Here's how the part is built. I have some questions about the finished solid (model axes, mm). Coordinates: 2 decimals unless noted, no trailing zeros. Write each loop counter-clockwise with the first axis right and the second up, starting at its lowest first coordinate (ties: lowest second). Pieces come first, ordered by that corner, then holes. Notation, with made-up numbers: (-2, 35) -> (41, 35) arc R23 ccw to (41, 47) -> close; hole circle Ø3 at (20, 64). An arc over 180 degrees is marked (long way). Put each result on its own line as item: value. Start each with the question number.
Item 1: I want a section at B-B, the plane x = 150. List the corners of the cut face in (y, z) for me, then the cut area to 3 significant figures.
Item 2: I want a section at A-A, the plane y = 94.5. List the corners of the cut face in (x, z) for me, then the cut area to 3 significant figures.
Item 3: I need wall thicknesses on line 1 (X direction, y = 254.5, z = 1); line 2 (X direction, y = 205, z = 5.25); line 3 (Y direction, x = -48, z = 0.5). Which ranges of each line are inside material? Lowest first, please. Write a range as [from, to].
Item 4: I want a section at C-C, the plane z = 10. State how many separate pieces and enclosed holes the cut face has, then the cut area to 3 significant figures.
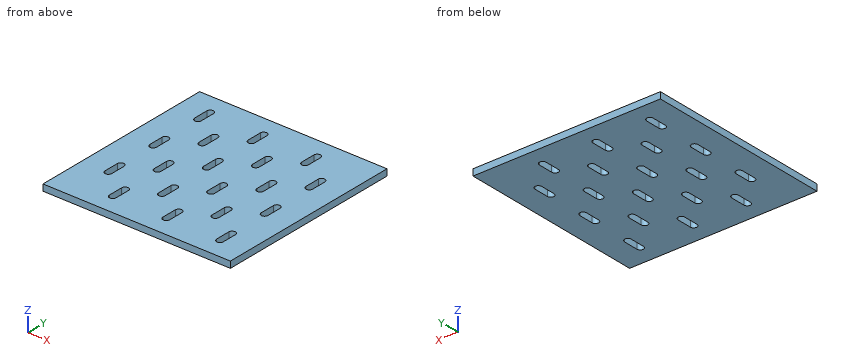
from build123d import *

# Parameters (mm, degrees)
SKETCH_1_W      = 350
SKETCH_1_H      = 350
EXTRUDE_1_DEPTH = 12


with BuildPart() as part:
    # Эскиз1 → Бобышка-Вытянуть1 (new body)
    with BuildSketch(Plane.XY):
        with Locations((75, 125)):
            Rectangle(SKETCH_1_W, SKETCH_1_H)
        with BuildLine():
            Line((6.25, 13.75), (6.25, -13.75))
            ThreePointArc((6.25, -13.75), (0, -20), (-6.25, -13.75))
            Line((-6.25, -13.75), (-6.25, 13.75))
            ThreePointArc((-6.25, 13.75), (0, 20), (6.25, 13.75))
        make_face(mode=Mode.SUBTRACT)
        with BuildLine():
            Line((-43.75, 63.75), (-43.75, 36.25))
            ThreePointArc((-43.75, 36.25), (-50, 30), (-56.25, 36.25))
            Line((-56.25, 36.25), (-56.25, 63.75))
            ThreePointArc((-56.25, 63.75), (-50, 70), (-43.75, 63.75))
        make_face(mode=Mode.SUBTRACT)
        with BuildLine():
            Line((106.25, 13.75), (106.25, -13.75))
            ThreePointArc((106.25, -13.75), (100, -20), (93.75, -13.75))
            Line((93.75, -13.75), (93.75, 13.75))
            ThreePointArc((93.75, 13.75), (100, 20), (106.25, 13.75))
        make_face(mode=Mode.SUBTRACT)
        with BuildLine():
            Line((56.25, 63.75), (56.25, 36.25))
            ThreePointArc((56.25, 36.25), (50, 30), (43.75, 36.25))
            Line((43.75, 36.25), (43.75, 63.75))
            ThreePointArc((43.75, 63.75), (50, 70), (56.25, 63.75))
        make_face(mode=Mode.SUBTRACT)
        with BuildLine():
            Line((206.25, 13.75), (206.25, -13.75))
            ThreePointArc((206.25, -13.75), (200, -20), (193.75, -13.75))
            Line((193.75, -13.75), (193.75, 13.75))
            ThreePointArc((193.75, 13.75), (200, 20), (206.25, 13.75))
        make_face(mode=Mode.SUBTRACT)
        with BuildLine():
            Line((156.25, 63.75), (156.25, 36.25))
            ThreePointArc((156.25, 36.25), (150, 30), (143.75, 36.25))
            Line((143.75, 36.25), (143.75, 63.75))
            ThreePointArc((143.75, 63.75), (150, 70), (156.25, 63.75))
        make_face(mode=Mode.SUBTRACT)
        with BuildLine():
            Line((106.25, 113.75), (106.25, 86.25))
            ThreePointArc((106.25, 86.25), (100, 80), (93.75, 86.25))
            Line((93.75, 86.25), (93.75, 113.75))
            ThreePointArc((93.75, 113.75), (100, 120), (106.25, 113.75))
        make_face(mode=Mode.SUBTRACT)
        with BuildLine():
            Line((56.25, 163.75), (56.25, 136.25))
            ThreePointArc((56.25, 136.25), (50, 130), (43.75, 136.25))
            Line((43.75, 136.25), (43.75, 163.75))
            ThreePointArc((43.75, 163.75), (50, 170), (56.25, 163.75))
        make_face(mode=Mode.SUBTRACT)
        with BuildLine():
            Line((206.25, 113.75), (206.25, 86.25))
            ThreePointArc((206.25, 86.25), (200, 80), (193.75, 86.25))
            Line((193.75, 86.25), (193.75, 113.75))
            ThreePointArc((193.75, 113.75), (200, 120), (206.25, 113.75))
        make_face(mode=Mode.SUBTRACT)
        with BuildLine():
            Line((156.25, 163.75), (156.25, 136.25))
            ThreePointArc((156.25, 136.25), (150, 130), (143.75, 136.25))
            Line((143.75, 136.25), (143.75, 163.75))
            ThreePointArc((143.75, 163.75), (150, 170), (156.25, 163.75))
        make_face(mode=Mode.SUBTRACT)
        with BuildLine():
            Line((106.25, 213.75), (106.25, 186.25))
            ThreePointArc((106.25, 186.25), (100, 180), (93.75, 186.25))
            Line((93.75, 186.25), (93.75, 213.75))
            ThreePointArc((93.75, 213.75), (100, 220), (106.25, 213.75))
        make_face(mode=Mode.SUBTRACT)
        with BuildLine():
            Line((56.25, 263.75), (56.25, 236.25))
            ThreePointArc((56.25, 236.25), (50, 230), (43.75, 236.25))
            Line((43.75, 236.25), (43.75, 263.75))
            ThreePointArc((43.75, 263.75), (50, 270), (56.25, 263.75))
        make_face(mode=Mode.SUBTRACT)
        with BuildLine():
            Line((206.25, 213.75), (206.25, 186.25))
            ThreePointArc((206.25, 186.25), (200, 180), (193.75, 186.25))
            Line((193.75, 186.25), (193.75, 213.75))
            ThreePointArc((193.75, 213.75), (200, 220), (206.25, 213.75))
        make_face(mode=Mode.SUBTRACT)
        with BuildLine():
            Line((156.25, 263.75), (156.25, 236.25))
            ThreePointArc((156.25, 236.25), (150, 230), (143.75, 236.25))
            Line((143.75, 236.25), (143.75, 263.75))
            ThreePointArc((143.75, 263.75), (150, 270), (156.25, 263.75))
        make_face(mode=Mode.SUBTRACT)
        with BuildLine():
            Line((6.25, 113.75), (6.25, 86.25))
            ThreePointArc((6.25, 86.25), (0, 80), (-6.25, 86.25))
            Line((-6.25, 86.25), (-6.25, 113.75))
            ThreePointArc((-6.25, 113.75), (0, 120), (6.25, 113.75))
        make_face(mode=Mode.SUBTRACT)
        with BuildLine():
            Line((-43.75, 163.75), (-43.75, 136.25))
            ThreePointArc((-43.75, 136.25), (-50, 130), (-56.25, 136.25))
            Line((-56.25, 136.25), (-56.25, 163.75))
            ThreePointArc((-56.25, 163.75), (-50, 170), (-43.75, 163.75))
        make_face(mode=Mode.SUBTRACT)
        with BuildLine():
            Line((6.25, 213.75), (6.25, 186.25))
            ThreePointArc((6.25, 186.25), (0, 180), (-6.25, 186.25))
            Line((-6.25, 186.25), (-6.25, 213.75))
            ThreePointArc((-6.25, 213.75), (0, 220), (6.25, 213.75))
        make_face(mode=Mode.SUBTRACT)
        with BuildLine():
            Line((-43.75, 263.75), (-43.75, 236.25))
            ThreePointArc((-43.75, 236.25), (-50, 230), (-56.25, 236.25))
            Line((-56.25, 236.25), (-56.25, 263.75))
            ThreePointArc((-56.25, 263.75), (-50, 270), (-43.75, 263.75))
        make_face(mode=Mode.SUBTRACT)
    extrude(amount=EXTRUDE_1_DEPTH)


solid = part.part
Calculated:
1. outline: (-50, 0) -> (30, 0) -> (30, 12) -> (-50, 12) -> close; (70, 0) -> (130, 0) -> (130, 12) -> (70, 12) -> close; (170, 0) -> (230, 0) -> (230, 12) -> (170, 12) -> close; (270, 0) -> (300, 0) -> (300, 12) -> (270, 12) -> close
1. area: 2,760 mm2
2. outline: (-100, 0) -> (-6.25, 0) -> (-6.25, 12) -> (-100, 12) -> close; (6.25, 0) -> (93.75, 0) -> (93.75, 12) -> (6.25, 12) -> close; (106.25, 0) -> (193.75, 0) -> (193.75, 12) -> (106.25, 12) -> close; (206.25, 0) -> (250, 0) -> (250, 12) -> (206.25, 12) -> close
2. area: 3,750 mm2
3. line 1: x = [-100, -56.25], [-43.75, 43.75], [56.25, 143.75], [156.25, 250]
3. line 2: x = [-100, -6.25], [6.25, 93.75], [106.25, 193.75], [206.25, 250]
3. line 3: y = [-50, 30.33], [69.67, 130.33], [169.67, 230.33], [269.67, 300]
4. separate pieces: 1
4. enclosed holes: 18
4. area: 114,000 mm2
